For this review, take the finished solid that the model builds, in its own axes (mm). A direction names the side the tool comes from. Coordinates: 2 decimals unless noted, no trailing zeros. Use one line per item in the form item = value. Start each with the question number.
1) Insertion check: P1, Ø7, axis at x = -5.5, z = -20, coming from the -Y side. The pin has a flat end and moves straight along its axis. Give the tip position at first contact, or say it passes through.
2) Mouldability with a two-part tool opening along X and no side actions: class faces 3 (the cylindrical face through (-8.01, -107.913, -26.746)), 4 (the flat face through (11.838, -115.791, 2.322)), 5 (the flat face through (-25.66, -115.79, -23.55)) as pulls with the +X half, pulls with the -X half, needs draft (parallel to the pull), parting line crosses it, or undercut.
3) For L1, parallel to Z at x = -6, y = -105.5; L2, parallel to Y at x = -12, z = -19.5; L3, parallel to Y at x = -2.5, z = -21, list the stretches that pass through material, from the lowest coordinate up. Write a range as from..to.
4) Tool access review of faces 1 (the flat face through (-1, -110.295, -23)), 2 (the flat face through (12, -118.295, -23)): name each direction out of +Z, -Z, +X, -X, +Y, -Y from which nothing blocks a thin tool from reaching the whole face with its end or side.
```python
from build123d import *

# Parameters (mm, degrees)
F0_W           = 81.2892764807
F0_H           = 56.1117217876
F1_DEPTH       = 118.29543
F3_D           = 8.8
F3_DEPTH       = 12.7
F3_CBORE_D     = 14.25
F3_CBORE_DEPTH = 8
F3_TIP         = 2.6437867237
F4_SIZE        = 5.08


with BuildPart() as f1:
    # F0 (on Front) → F1 (new body)
    with BuildSketch(Plane.XZ):
        with Locations((12.407310307, -23.1582082342)):
            Rectangle(F0_W, F0_H)
    extrude(amount=F1_DEPTH)

    # F3
    with Locations(Plane.XZ.offset(118.29543)):
        with Locations((-5.9798196889, -22.842913866)):
            CounterBoreHole(F3_D / 2, F3_CBORE_D / 2, F3_CBORE_DEPTH, depth=F3_DEPTH)
            with Locations((0, 0, -(F3_DEPTH + F3_TIP / 2))):  # 118° drill point
                Cone(0, F3_D / 2, F3_TIP, mode=Mode.SUBTRACT)

    # F4
    f4_edges = [f1.edges().sort_by_distance(p)[0] for p in [
        (12.40731, -118.29543, 4.897653),
        (53.051949, -118.29543, -23.158208),
        (-28.237328, -118.29543, -23.158208),
        (12.40731, -118.29543, -51.214069),
        (-13.10482, -118.29543, -22.842914),
    ]]
    chamfer(f4_edges, length=F4_SIZE)


solid = f1.part
```
Determined:
q1.P1 = -110.3
q2.face_3 = undercut
q2.face_4 = needs draft
q2.face_5 = pulls with the -X half
q3.L1 = -51.21..-27.08, -18.6..4.9
q3.L2 = -110.3..0
q3.L3 = -105.32..0
q4.face_1 = -Y
q4.face_2 = +Z, -Z, +X, -X, -Y
